from build123d import *

# Parameters (mm, degrees)
F0_W     = 145
F0_H     = 125
F0_W_2   = 125
F0_H_2   = 105
F1_DEPTH = 1
F2_R     = 5
F4_DEPTH = 25


with BuildPart() as f1:
    # F0 (on Top) → F1 (new body)
    with BuildSketch(Plane.XY):
        Rectangle(F0_W, F0_H)
        Rectangle(F0_W_2, F0_H_2, mode=Mode.SUBTRACT)
    extrude(amount=F1_DEPTH)

    # F2
    f2_edges = [f1.edges().sort_by_distance(p)[0] for p in [
        (-62.5, 52.5, 0.5),
        (-62.5, -52.5, 0.5),
        (62.5, -52.5, 0.5),
        (62.5, 52.5, 0.5),
    ]]
    fillet(f2_edges, radius=F2_R)

    # F3 (on face) → F4 (join)
    with BuildSketch(Plane.XY.offset(1)):
        with BuildLine():
            ThreePointArc((-57.5, 53.500002), (-61.742642, 51.742642), (-63.500002, 47.5))
            Line((-63.500002, 47.5), (-63.500002, -47.5))
            ThreePointArc((-63.500002, -47.5), (-61.742642, -51.742642), (-57.5, -53.500002))
            Line((-57.5, -53.500002), (57.5, -53.500002))
            ThreePointArc((57.5, -53.500002), (61.742642, -51.742642), (63.500002, -47.5))
            Line((63.500002, -47.5), (63.500002, 47.5))
            ThreePointArc((63.500002, 47.5), (61.742642, 51.742642), (57.5, 53.500002))
            Line((57.5, 53.500002), (-57.5, 53.500002))
        make_face()
        with BuildLine():
            ThreePointArc((-57.5, -52.5), (-61.035534, -51.035534), (-62.5, -47.5))
            Line((-62.5, -47.5), (-62.5, 47.5))
            ThreePointArc((-62.5, 47.5), (-61.035534, 51.035534), (-57.5, 52.5))
            Line((-57.5, 52.5), (57.5, 52.5))
            ThreePointArc((57.5, 52.5), (61.035534, 51.035534), (62.5, 47.5))
            Line((62.5, 47.5), (62.5, -47.5))
            ThreePointArc((62.5, -47.5), (61.035534, -51.035534), (57.5, -52.5))
            Line((57.5, -52.5), (-57.5, -52.5))
        make_face(mode=Mode.SUBTRACT)
    extrude(amount=-F4_DEPTH)


solid = f1.part
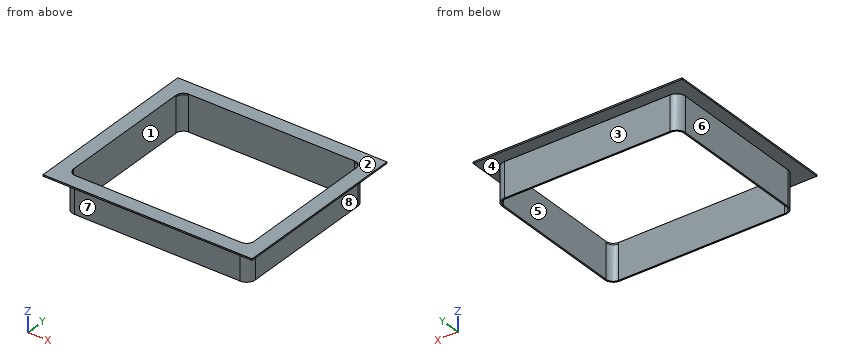
The listing builds one solid part. Answer for the finished solid, in the listing's coordinates (mm). Face numbers are marked on the shaded views. A direction names the side the tool comes from. Coordinates: 2 decimals unless noted, no trailing zeros. Write each loop counter-clockwise with the first axis right and the second up, starting at its lowest first coordinate (ties: lowest second). Pieces come first, ordered by that corner, then holes. Notation, with made-up numbers: M 22.5,-7.5 L 49.5,-7.5 A23 cw 49.5,22.5 Z; hole C -25.75,39 d5. An arc over 180 degrees is marked long. Write each question's results on one line, items separated by ' | '.
Item 1: The part is cut by section B-B on x = 24. Determine the outline of the cut face in (y, z), and give its area (3 significant figures).
Answer below:
outline: M -62.5,0 L -53.5,0 L -53.5,-24 L -52.5,-24 L -52.5,1 L -62.5,1 Z; M 52.5,-24 L 53.5,-24 L 53.5,0 L 62.5,0 L 62.5,1 L 52.5,1 Z | area: 68.0 mm2
Item 2: Given P1, Ø1.5, axis at x = 42.5, z = -6.5, coming from the +Y side; P2, Ø7.5, axis at y = 18.5, z = -10.5, coming from the -X side; P3, Ø3, axis at y = -48, z = -2, coming from the +X side, each flat-ended and moving along its own axis, determine where each tip first touches the part or whether it passes through.
Answer below:
P1: y = 53.5 | P2: x = -63.5 | P3: x = 63.5
Item 3: Consider probe 1 along Y at (x, z) = (13, -11.5); probe 2 along X at (y, z) = (12, -2); probe 3 along Z at (x, y) = (-64, 30.5). Determine where each line is inside the solid, lowest interval first. Write a range as [from, to].
Answer below:
probe 1: [-53.5, -52.5], [52.5, 53.5] | probe 2: [-63.5, -62.5], [62.5, 63.5] | probe 3: [0, 1]
Item 4: For a pull along X with two mould halves and no side action, classify the marked faces 5, 6, 7 and 8 as released by +X, released by -X, zero draft, split by the parting line, or undercut.
Answer below:
face 5: undercut | face 6: released by -X | face 7: zero draft | face 8: released by +X
Item 5: The part is cut by section A-A on y = -0.5. Determine the outline of the cut face in (x, z), and give its area (3 significant figures).
Answer below:
outline: M -72.5,0 L -63.5,0 L -63.5,-24 L -62.5,-24 L -62.5,1 L -72.5,1 Z; M 62.5,-24 L 63.5,-24 L 63.5,0 L 72.5,0 L 72.5,1 L 62.5,1 Z | area: 68.0 mm2
Item 6: The part is cut by section C-C on z = -6.5. Determine the outline of the cut face in (x, y).
Answer below:
outline: M -63.5,-47.5 A6 ccw -57.5,-53.5 L 57.5,-53.5 A6 ccw 63.5,-47.5 L 63.5,47.5 A6 ccw 57.5,53.5 L -57.5,53.5 A6 ccw -63.5,47.5 Z; hole M -62.5,-47.5 A5 ccw -57.5,-52.5 L 57.5,-52.5 A5 ccw 62.5,-47.5 L 62.5,47.5 A5 ccw 57.5,52.5 L -57.5,52.5 A5 ccw -62.5,47.5 Z
Item 7: Which of the six approach directions +Z, -Z, +X, -X, +Y, -Y give full straight-line access (tool end or side, diameter ignored) to the marked faces 1, 2, 3 and 4?
Answer below:
face 1: +Z, -Z | face 2: +Z, +X, -X, +Y, -Y | face 3: -Z, +X, -X, +Y | face 4: -Z
